Could you check a few things on this model? Use its own coordinates, in mm. A direction names the side the tool comes from. Give positions to 0.01 mm unless a question says otherwise; leave off trailing zeros. Loops run counter-clockwise (first coordinate to the right, second up) from the corner with the lowest first, then second, coordinate; pieces in that order, holes last. Notation, with made-up numbers: M 15,-31 L 60,-31 A19 ccw 60,-12 Z; hole C 81.25,2.5 d1. An arc over 180 degrees is marked long. Use CSV: the item, a comma, the result in double quotes.
```python
from build123d import *

# Parameters (mm, degrees)
ESQUISSE1_R             = 11
BOSS_EXTRU_1_DEPTH      = 7.5
ESQUISSE3_R             = 15
BOSS_EXTRU_2_DEPTH      = 6.5
CHANFREIN1_SIZE         = 0.5
CHANFREIN2_SIZE         = 1
ESQUISSE4_R             = 14.5
ENL_V_MAT_EXTRU_1_DEPTH = 3.5
ESQUISSE5_R             = 4.5
ENL_V_MAT_EXTRU_2_DEPTH = 1.5
ESQUISSE6_R             = 7
ENL_V_MAT_EXTRU_3_DEPTH = 1
ESQUISSE8_R             = 8
ENL_V_MAT_EXTRU_4_DEPTH = 23.671568098


with BuildPart() as part:
    # Esquisse1 → Boss.-Extru.1 (new body)
    with BuildSketch(Plane(origin=(0, 0, 0), x_dir=(1, 0, 0), z_dir=(0, 1, 0))):
        with Locations(Location((0, 0, 0), (0, 0, 270))):
            Circle(ESQUISSE1_R)
    extrude(amount=BOSS_EXTRU_1_DEPTH)

    # Esquisse3 → Boss.-Extru.2 (add)
    with BuildSketch(Plane(origin=(0, 7.5, 0), x_dir=(1, 0, 0), z_dir=(0, 1, 0))):
        with Locations(Location((0, 0, 0), (0, 0, 90))):
            Circle(ESQUISSE3_R)
    extrude(amount=BOSS_EXTRU_2_DEPTH)

    # Chanfrein1
    chanfrein1_edges = [part.edges().sort_by_distance(p)[0] for p in [
        (0, 0, -11),
    ]]
    chamfer(chanfrein1_edges, length=CHANFREIN1_SIZE)

    # Chanfrein2
    chanfrein2_edges = [part.edges().sort_by_distance(p)[0] for p in [
        (0, 7.5, -11),
    ]]
    chamfer(chanfrein2_edges, length=CHANFREIN2_SIZE)

    # Esquisse4 → Enlèv. mat.-Extru.1 (cut)
    with BuildSketch(Plane(origin=(0, 14, 0), x_dir=(1, 0, 0), z_dir=(0, 1, 0))):
        with Locations(Location((0, 0, 0), (0, 0, 270))):
            Circle(ESQUISSE4_R)
    extrude(amount=-ENL_V_MAT_EXTRU_1_DEPTH, mode=Mode.SUBTRACT)

    # Esquisse5 → Enlèv. mat.-Extru.2 (cut)
    with BuildSketch(Plane(origin=(0, 10.5, 0), x_dir=(1, 0, 0), z_dir=(0, 1, 0))):
        with Locations(Location((0, 0, 0), (0, 0, 270))):
            Circle(ESQUISSE5_R)
    extrude(amount=-ENL_V_MAT_EXTRU_2_DEPTH, mode=Mode.SUBTRACT)

    # Esquisse6 → Enlèv. mat.-Extru.3 (cut)
    with BuildSketch(Plane(origin=(0, 9, 0), x_dir=(1, 0, 0), z_dir=(0, 1, 0))):
        with Locations(Location((0, 0, 0), (0, 0, 270))):
            Circle(ESQUISSE6_R)
    extrude(amount=-ENL_V_MAT_EXTRU_3_DEPTH, mode=Mode.SUBTRACT)

    # Esquisse8 → Enlèv. mat.-Extru.4 (cut, through all)
    with BuildSketch(Plane(origin=(0, 8, 0), x_dir=(1, 0, 0), z_dir=(0, 1, 0))):
        with Locations(Location((0, 0, 0), (0, 0, 270))):
            Circle(ESQUISSE8_R)
    extrude(amount=-ENL_V_MAT_EXTRU_4_DEPTH, mode=Mode.SUBTRACT)


solid = part.part
```
1. Please list where these lines run through material, in increasing order: line 1 (X direction, y = 3.75, z = 0); line 2 (X direction, y = 9.85, z = 0); line 3 (Y direction, x = -12, z = 7.25).
Outcome:
line 1,"-11 to -8, 8 to 11"
line 2,"-15 to -4.5, 4.5 to 15"
line 3,"7.5 to 10.5"
2. I want a section at D-D, the plane y = 3.25. List the corners of the cut face in (x, z) for me.
Outcome:
outline,"C 0,0 d22; hole C 0,0 d16"
3. I want a section at C-C, the plane y = 10. List the corners of the cut face in (x, z) for me.
Outcome:
outline,"C 0,0 d30; hole C 0,0 d9"
4. I want a section at A-A, the plane z = 0. List the corners of the cut face in (x, y) for me.
Outcome:
outline,"M -15,7.5 L -12,7.5 L -11,6.5 L -11,0.5 L -10.5,0 L -8,0 L -8,8 L -7,8 L -7,9 L -4.5,9 L -4.5,10.5 L -14.5,10.5 L -14.5,14 L -15,14 Z; M 4.5,9 L 7,9 L 7,8 L 8,8 L 8,0 L 10.5,0 L 11,0.5 L 11,6.5 L 12,7.5 L 15,7.5 L 15,14 L 14.5,14 L 14.5,10.5 L 4.5,10.5 Z"
5. I'm going to push flat-ended pins straight in: pin 1 Ø4 at (x, y) = (-7, 6) entering from +Z; pin 2 Ø6 at (y, z) = (7.5, -4.5) entering from +X; pin 3 Ø12.5 at (x, z) = (0, 0) entering from +Y. Where does each tip first touch, or does it pass through?
Outcome:
pin 1,"z = 13.88"
pin 2,"x = 14.92"
pin 3,"y = 10.5"
6. If we mould it in two halves opening along X, with no side actions, what happens to faces 4 (the face through (-8, 0, -2)), 5 (the face through (-0.66, 10.704, 14.985)), 6 (the face through (-5.554, 12.274, 13.394))? For each: +X half, -X half, draft (parallel to the pull), parting line (faces both ways), or undercut.
Outcome:
face 4,"draft"
face 5,"parting line"
face 6,"undercut"
7. I want a section at B-B, the plane x = 0. List the corners of the cut face in (y, z) for me.
Outcome:
outline,"M 0,-10.5 L 0.5,-11 L 6.5,-11 L 7.5,-12 L 7.5,-15 L 14,-15 L 14,-14.5 L 10.5,-14.5 L 10.5,-4.5 L 9,-4.5 L 9,-7 L 8,-7 L 8,-8 L 0,-8 Z; M 0,8 L 8,8 L 8,7 L 9,7 L 9,4.5 L 10.5,4.5 L 10.5,14.5 L 14,14.5 L 14,15 L 7.5,15 L 7.5,12 L 6.5,11 L 0.5,11 L 0,10.5 Z"
8. Which directions (+Z, -Z, +X, -X, +Y, -Y) give clear straight access to the entire face, cutting with the end or side of a thin tool? Please do faces 1 (the face through (1.352, 9.76, 4.292)), 2 (the face through (-7.81, 4.06, -1.73)), 3 (the face through (3.4, 10.5, -3.4)).
Outcome:
face 1,"+Y, -Y"
face 2,"-Y"
face 3,"+Y"
